Autodesk Inventor part; units mm, degrees
ref_plane "YZ Plane" through (0, 0, 0) normal (1, 0, 0) x (0, 1, 0)
ref_plane "XZ Plane" through (0, 0, 0) normal (0, 1, 0) x (-1, 0, 0)
ref_plane "XY Plane" through (0, 0, 0) normal (0, 0, 1) x (1, 0, 0)
sketch "Sketch1" plane through (0, 0, 0) normal (0, 0, 1) x (1, 0, 0)
  line L0 (-9.1, 0) -> (9.1, 0) construction
  line L1 (0, -6.0044) -> (0, 9.7572) construction
  line L2 (0, 7.5056) -> (6.5, -3.7528)
  line L3 (6.5, -3.7528) -> (-6.5, -3.7528)
  line L4 (-6.5, -3.7528) -> (0, 7.5056)
  point P0 (0, 0)
  point P1 (0, 0)
  dimension "d0" = 13
extrude "Extrusion1" add sketch "Sketch1" along normal blind 0.4
fillet "Fillet1" radius 1 3 edges at (-6.5, -3.7528, 0.2) (6.5, -3.7528, 0.2) (0, 7.5056, 0.2)
sketch "Sketch2" plane through (0, 0, 0.4) normal (0, 0, 1) x (1, 0, 0)
  arc A0 (-5.634, -2.2528) -> (-4.7679, -3.7528) centre (-4.7679, -2.7528) ccw
  line L0 (-5.634, -2.2528) -> (-0.866, 6.0056)
  arc A1 (0.866, 6.0056) -> (-0.866, 6.0056) centre (0, 5.5056) ccw
  line L1 (0.866, 6.0056) -> (5.634, -2.2528)
  arc A2 (4.7679, -3.7528) -> (5.634, -2.2528) centre (4.7679, -2.7528) ccw
  line L2 (4.7679, -3.7528) -> (-4.7679, -3.7528)
  line L3 (-0.1732, 5.6056) -> (-4.9412, -2.6528)
  arc A3 (-4.9412, -2.6528) -> (-4.7679, -2.9528) centre (-4.7679, -2.7528) ccw
  line L4 (-4.7679, -2.9528) -> (4.7679, -2.9528)
  arc A4 (4.7679, -2.9528) -> (4.9412, -2.6528) centre (4.7679, -2.7528) ccw
  line L5 (4.9412, -2.6528) -> (0.1732, 5.6056)
  arc A5 (0.1732, 5.6056) -> (-0.1732, 5.6056) centre (0, 5.5056) ccw
  circle A6 centre (0, 0) radius 1.25
  dimension "d4" = 0.8
  dimension "d5" = 2.5
extrude "Extrusion2" add sketch "Sketch2" along normal blind 0.4 contours A5 L5 A4 L4 A3 L3
sketch "Sketch3" plane through (0, 0, 0.8) normal (0, 0, 1) x (1, 0, 0)
  line L0 (-8.0751, 0) -> (8.0751, 0) construction
  line L1 (0, -5.8044) -> (0, 8.5572) construction
  circle A0 centre (0, 0) radius 1.25 construction
  line L2 (-0.15, 2.5) -> (0.15, 2.5)
  line L3 (0.15, 2.5) -> (0.15, -0.4687)
  line L4 (0.15, -0.4687) -> (-0.15, -0.4687)
  line L5 (-0.15, -0.4687) -> (-0.15, 2.5)
  point P0 (0, 2.5)
  dimension "d8" = 0.3
  dimension "d9" = 2.5
extrude "Extrusion3" cut sketch "Sketch3" against normal blind 0.4
pattern_circular "Circular Pattern1" count 8 over 360 about axis through (0, 0, -10) along (0, 0, 1) of "Extrusion3"
sketch "Sketch4" plane through (0, 0, 0.8) normal (0, 0, 1) x (1, 0, 0)
  line L0 (0, -5.8044) -> (0, 8.5572) construction
  line L1 (-8.0751, 0) -> (8.0751, 0) construction
  line L2 (0, 0) -> (1.8051, 4.3579) construction
  line L3 (0.6268, 1.9052) -> (0.9039, 1.7904)
  line L4 (0.9039, 1.7904) -> (0.2506, 0.2129)
  line L5 (0.2506, 0.2129) -> (-0.0266, 0.3277)
  line L6 (-0.0266, 0.3277) -> (0.6268, 1.9052)
  point P0 (0.7654, 1.8478)
  dimension "d15" = 22.5
  dimension "d16" = 0.3
  dimension "d17" = 2
extrude "Extrusion4" cut sketch "Sketch4" against normal blind 0.4
pattern_circular "Circular Pattern2" count 8 over 360 about axis through (0, 0, -10) along (0, 0, 1) of "Extrusion4"
sketch "Sketch5" plane through (0, 0, 0.8) normal (0, 0, 1) x (1, 0, 0)
  line L0 (1.241, 0.15) -> (2.5, 0.15) construction
  line L1 (2.5, -0.15) -> (1.241, -0.15) construction
  line L2 (2.5, 0.15) -> (5.6384, 0.15)
  line L3 (5.6384, 0.15) -> (5.6384, -0.15)
  line L4 (5.6384, -0.15) -> (2.5, -0.15)
  line L5 (2.5, -0.15) -> (2.5, 0.15)
  point P0 (0, 0)
extrude "Extrusion5" cut sketch "Sketch5" against normal blind 0.4
properties part number "P129"
Verification items for the finished model (mm, model axes). A direction names the side the tool comes from. Coordinates: 2 decimals unless noted, no trailing zeros. Order: outer loops, then holes, each group sorted by start corner. A loop starts at its lowest first (then second) coordinate and runs counter-clockwise, first axis right, second up. Notation, with made-up numbers: (85, 6) -> (144, 6) arc R16 ccw to (144, 14) -> close; hole circle Ø6 at (-32.5, 74.5). An arc over 180 degrees is marked (long way). Answer as CSV lines item,"result". Start each with the question number.
1) Set-up check for faces 1 (the face through (1.43, 1.22, 0.6)), 2 (the face through (5.627, -3.265, 0.203)), 3 (the face through (4.23, -1.42, 0.6)): record each of +Z, -Z, +X, -X, +Y, -Y from which the full face is reachable in a straight line by a thin tool's end or side.
2) Gauge pin test, flat end, axial feed: pin 1 Ø5 at (x, y) = (-4.5, 2) entering from -Z. Record the tip position at first contact, or that the pin passes through.
3) Cross-section at C-C, the plane y = 3. Record the boundary of the cut face in (x, z), then the cut area to 3 significant figures.
4) Cross-section at B-B, the plane z = 0.15. Record the boundary of the cut face in (x, y).
5) Material ranges on L1, parallel to X at y = 0.75, z = 0.55; L2, parallel to Z at x = -3.5, y = -3; L3, parallel to X at y = -2.75, z = 0.55, recorded low to high. Write a range as [from, to].
6) Cross-section at A-A, the plane x = -3.25. Record the boundary of the cut face in (y, z).
7) Release check for a two-part mould opening along X. For faces 4 (the face through (1.22, -1.43, 0.6)), 5 (the face through (-2.524, 1.534, 0.597)), 6 (the face through (3.22, 1.93, 0.2)), 7 (the face through (1.21, 1.42, 0.6)) record: released by +X, released by -X, zero draft, split by the parting line, or undercut.
8) Cross-section at D-D, the plane x = 5.25. Record the boundary of the cut face in (y, z).
Conclusion:
1,face 1,"+Z"
1,face 2,"+Z, -Z, +X"
1,face 3,"+Z, +X, +Y"
2,pin 1,"stops at z = 0"
3,outline,"(-2.6, 0) -> (2.6, 0) -> (2.6, 0.4) -> (1.68, 0.4) -> (1.68, 0.8) -> (-1.68, 0.8) -> (-1.68, 0.4) -> (-2.6, 0.4) -> close"
3,area,"3.42 mm²"
4,outline,"(-5.63, -2.25) arc R1 ccw to (-4.77, -3.75) -> (4.77, -3.75) arc R1 ccw to (5.63, -2.25) -> (0.87, 6.01) arc R1 ccw to (-0.87, 6.01) -> close"
5,L1,"x = [-2.98, -1.85], [-1.42, -1], [1, 1.42], [1.85, 2.98]"
5,L2,"z = [0, 0.4]"
5,L3,"x = [-4.97, 4.97]"
6,outline,"(-3.75, 0) -> (1.88, 0) -> (1.88, 0.4) -> (0.28, 0.4) -> (0.28, 0.8) -> (-2.95, 0.8) -> (-2.95, 0.4) -> (-3.75, 0.4) -> close"
7,face 4,"undercut"
7,face 5,"released by -X"
7,face 6,"released by +X"
7,face 7,"undercut"
8,outline,"(-3.63, 0) -> (-1.59, 0) -> (-1.59, 0.4) -> (-3.63, 0.4) -> close"
